Can you work these out from the model? Positions are in its coordinate system, mm. Face numbers are marked on the shaded views. Round coordinates to 2 decimals unless told otherwise and drop trailing zeros. Order: outer loops, then holes, each group sorted by start corner. A loop starts at its lowest first (then second) coordinate and runs counter-clockwise, first axis right, second up. Notation, with made-up numbers: M -38,-5.5 L -7,-5.5 A9 cw -7,11.5 Z; hole C 31,72 d9. An arc over 180 degrees is marked long. One line per question, with ' | ' between items.
```python
from build123d import *

# Parameters (mm, degrees)
BOSS_EXTRUDE1_DEPTH = 200
SKETCH2_W           = 110
SKETCH2_H           = 25
CUT_EXTRUDE1_DEPTH  = 50
BOSS_EXTRUDE2_DEPTH = 15


with BuildPart() as part:
    # Sketch1 → Boss-Extrude1 (new body)
    with BuildSketch(Plane.XY):
        Polygon((115, 90), (115, 100), (120, 100), (120, 90), (120, 85.000009832), (120, 5.000009832), (120, 0), (0, 0), (0, 5), (0, 85), (0, 90), (0, 100), (5, 100), (5, 90), align=None)
        Polygon((115, 45.000009832), (115, 50.000009832), (115, 85.000009832), (5, 85.000009832), (5, 50.000009832), (5, 45.000009832), (5, 5.000009832), (115, 5.000009832), align=None, mode=Mode.SUBTRACT)
    extrude(amount=-BOSS_EXTRUDE1_DEPTH)

    # Sketch2 → Cut-Extrude1 (cut)
    with BuildSketch(Plane(origin=(0, 90, 0), x_dir=(1, 0, 0), z_dir=(0, 1, 0))):
        with Locations((60, 184.5)):
            Rectangle(SKETCH2_W, SKETCH2_H)
        with Locations((60, 156.5)):
            Rectangle(SKETCH2_W, SKETCH2_H)
        with Locations((60, 128.5)):
            Rectangle(SKETCH2_W, SKETCH2_H)
        with Locations((60, 100.5)):
            Rectangle(SKETCH2_W, SKETCH2_H)
        with Locations((60, 72.5)):
            Rectangle(SKETCH2_W, SKETCH2_H)
        with Locations((60, 44.5)):
            Rectangle(SKETCH2_W, SKETCH2_H)
        with Locations((60, 16.5)):
            Rectangle(SKETCH2_W, SKETCH2_H)
        with Locations((60, -11.5)):
            Rectangle(SKETCH2_W, SKETCH2_H)
    extrude(amount=-CUT_EXTRUDE1_DEPTH, mode=Mode.SUBTRACT)

    # Sketch3 → Boss-Extrude2 (add)
    with BuildSketch(Plane.XY):
        Polygon((0, 100), (10, 100), (10, 5.000009832), (110, 5.000009832), (110, 100), (120, 100), (120, 0), (0, 0), align=None)
    extrude(amount=BOSS_EXTRUDE2_DEPTH)


solid = part.part
```
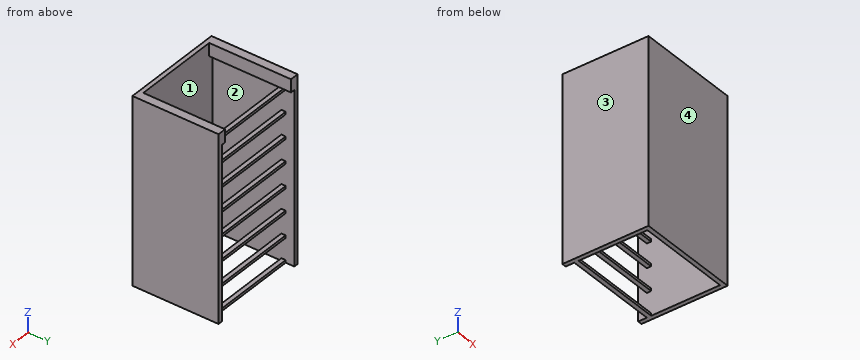
(1) If we section it at C-C on x = 90.5: State how many separate pieces and enclosed holes the cut face has, plus the area to 4 significant figures.
Final values:
separate pieces: 9 | enclosed holes: 0 | area: 1,195 mm^2
(2) Will these pins go through, and if not, where does the flat tip stop? pin 1 Ø6 at (x, z) = (93, -81) entering from +Y; pin 2 Ø1.5 at (x, z) = (34, -171) entering from +Y; pin 3 Ø3 at (x, z) = (91.5, -148.5) entering from -Y; pin 4 Ø4 at (x, y) = (74, 87) entering from +Z.
Final values:
pin 1: y = 5 | pin 2: y = 90 | pin 3: y = 0 | pin 4: z = -1
(3) If we section it at B-B on z = -72: Please give me the cut outline in (x, y), plus the area to 3 significant figures.
Final values:
outline: M 0,0 L 120,0 L 120,100 L 115,100 L 115,5 L 5,5 L 5,100 L 0,100 Z | area: 1,550 mm^2
(4) Thinking about a two-plate mould opening in X: for the marked faces 1, 2, 3 and 4, which applies, released by +X, released by -X, zero draft, split by the parting line, or undercut?
Final values:
face 1: undercut | face 2: undercut | face 3: released by -X | face 4: zero draft
(5) Please list where these lines run through material, in increasing order: probe 1 along X at (y, z) = (81, -173); probe 2 along Y at (x, z) = (106, -30.5); probe 3 along Y at (x, z) = (20, -47). Write a range as [from, to].
Final values:
probe 1: [0, 5], [115, 120] | probe 2: [0, 5], [85, 90] | probe 3: [0, 5]
(6) If we section it at A-A on y = 72: Please give me the cut outline in (x, z), plus the area to 3 significant figures.
Final values:
outline: M 0,-200 L 5,-200 L 5,0 L 10,0 L 10,15 L 0,15 Z; M 110,0 L 115,0 L 115,-200 L 120,-200 L 120,15 L 110,15 Z | area: 2,300 mm^2
